Verification items for the finished model (mm, model axes). A direction names the side the tool comes from. Coordinates: 2 decimals unless noted, no trailing zeros. Order: outer loops, then holes, each group sorted by start corner. A loop starts at its lowest first (then second) coordinate and runs counter-clockwise, first axis right, second up. Notation, with made-up numbers: M 48,22.25 L 90,22.25 A21 ccw 90,43.25 Z; hole C 81.5,79.5 d3. An arc over 180 degrees is marked long. Return JSON: item names as keys, results as strings.
```python
from build123d import *

# Parameters (mm, degrees)
SKETCH1_R           = 5
BOSS_EXTRUDE1_DEPTH = 20
BOSS_EXTRUDE2_DEPTH = 20
SKETCH6_W           = 95
SKETCH6_H           = 20
BOSS_EXTRUDE3_DEPTH = 115


with BuildPart() as part:
    # Sketch1 → Boss-Extrude1 (new body)
    with BuildSketch(Plane.XY):
        with BuildLine():
            Line((-67.5, -135), (-67.5, 0))
            ThreePointArc((-67.5, 0), (0, 67.5), (67.5, 0))
            Line((67.5, 0), (67.5, -135))
            Line((67.5, -135), (-67.5, -135))
        make_face()
        Circle(SKETCH1_R, mode=Mode.SUBTRACT)
    extrude(amount=BOSS_EXTRUDE1_DEPTH)

    # Sketch5 → Boss-Extrude2 (add)
    with BuildSketch(Plane(origin=(67.5, 0, 0), x_dir=(0, 0, -1), z_dir=(1, 0, 0))):
        Polygon((-20, 0), (-135, -115), (-135, -135), (-20, -135), align=None)
    boss_extrude2 = extrude(amount=-BOSS_EXTRUDE2_DEPTH)

    # Mirror1: Boss-Extrude2 across plane
    add(boss_extrude2.mirror(Plane(origin=(0, 0, 0), x_dir=(0, 0, 1), z_dir=(1, 0, 0))))

    # Sketch6 → Boss-Extrude3 (add)
    with BuildSketch(Plane.XY.offset(20)):
        with Locations((0, -125)):
            Rectangle(SKETCH6_W, SKETCH6_H)
    extrude(amount=BOSS_EXTRUDE3_DEPTH)


solid = part.part
```
Q1. Material ranges on line 1 along Y through (x, z) = (0, 8); line 2 along X through (y, z) = (-30, 46.5); line 3 along Y through (x, z) = (0, 28), recorded low to high.
Values:
{"line 1": "-135 to -5, 5 to 67.5", "line 2": "-67.5 to -47.5, 47.5 to 67.5", "line 3": "-135 to -115"}
Q2. Draft check along X on faces 1 (the face through (-67.5, -82, 53)), 2 (the face through (-58, -57, 77)), 3 (the face through (-47.5, -82, 53)). Enter one of: pulls with the +X half, pulls with the -X half, needs draft (parallel to the pull), parting line crosses it, or undercut.
Values:
{"face 1": "pulls with the -X half", "face 2": "needs draft", "face 3": "undercut"}
Q3. Go/stop test with flat-tipped pins: pin 1 (8 mm diameter, centred on x = -34, y = 3, fed in from +Z); pin 2 (3 mm diameter, centred on x = -50, y = -43.5, fed in from +Z). Record where each tip stops, or that it passes through.
Values:
{"pin 1": "z = 20", "pin 2": "z = 65"}
Q4. Cross-section at C-C, the plane y = -39. Record the boundary of the cut face in (x, z).
Values:
{"outline": "M -67.5,0 L 67.5,0 L 67.5,59 L 47.5,59 L 47.5,20 L -47.5,20 L -47.5,59 L -67.5,59 Z"}
Q5. Cross-section at A-A, the plane x = 0. Record the boundary of the cut face in (y, z), and give its area (3 significant figures).
Values:
{"outline": "M -135,0 L -5,0 L -5,20 L -115,20 L -115,135 L -135,135 Z; M 5,0 L 67.5,0 L 67.5,20 L 5,20 Z", "area": "6,150 mm^2"}
Q6. Tool access check on faces 4 (the face through (1, -22, 20)), 5 (the face through (-1, -125, 135)). Record the directions out of +Z, -Z, +X, -X, +Y, -Y that give a thin tool (end or side, any length) a straight path to the whole face; none if there is none.
Values:
{"face 4": "+Z, +Y", "face 5": "+Z, +X, -X, +Y, -Y"}
Q7. Cross-section at B-B, the plane z = 88. Record the boundary of the cut face in (x, y), and give its area (3 significant figures).
Values:
{"outline": "M -67.5,-135 L 67.5,-135 L 67.5,-68 L 47.5,-68 L 47.5,-115 L -47.5,-115 L -47.5,-68 L -67.5,-68 Z", "area": "4,580 mm^2"}
Q8. Cross-section at D-D, the plane x = -58. Record the boundary of the cut face in (y, z).
Values:
{"outline": "M -135,0 L 34.53,0 L 34.53,20 L 0,20 L -115,135 L -135,135 Z"}
